```python
from build123d import *

# Parameters (mm, degrees)
SKETCH009_W                   = 120
SKETCH009_H                   = 82
PAD002_DEPTH                  = 3
SKETCH010_W                   = 16.5
SKETCH010_H                   = 3
SKETCH010_W_2                 = 11
SKETCH010_W_3                 = 3
SKETCH010_H_2                 = 18
POCKET006_DEPTH               = 293.744874
SKETCH010_MIRRORED010_2_W     = 16.5
SKETCH010_MIRRORED010_2_H     = 3
SKETCH010_MIRRORED010_2_W_2   = 11
SKETCH010_MIRRORED010_2_W_3   = 3
SKETCH010_MIRRORED010_2_H_2   = 18
POCKET006_MIRRORED010_2_DEPTH = 293.744874
SKETCH011_W                   = 15
SKETCH011_H                   = 3
POCKET007_DEPTH               = 3.001
POCKET008_DEPTH               = 3.001
SKETCH013_W                   = 2.5
SKETCH013_H                   = 4
POCKET009_DEPTH               = 3.001


with BuildPart() as part:
    # Sketch009 → Pad002 (new body)
    with BuildSketch(Plane.XZ):
        Rectangle(SKETCH009_W, SKETCH009_H)
    extrude(amount=PAD002_DEPTH)

    # Sketch010 → Pocket006 (cut, through all)
    with BuildSketch(Plane.XZ):
        with Locations((-51.75, 39.5)):
            Rectangle(SKETCH010_W, SKETCH010_H)
        with Locations((-22, 39.5)):
            Rectangle(SKETCH010_W_2, SKETCH010_H)
        with Locations((0, 39.5)):
            Rectangle(SKETCH010_W_2, SKETCH010_H)
        with Locations((-58.5, 14.5)):
            Rectangle(SKETCH010_W_3, SKETCH010_H_2)
    pocket006 = extrude(amount=POCKET006_DEPTH, mode=Mode.SUBTRACT)

    # Sketch010 Mirrored010 2 → Pocket006 Mirrored010 2 (cut, through all)
    with BuildSketch(Plane(origin=(0, 0, 0), x_dir=(-1, 0, 0), z_dir=(0, 1, 0))):
        with Locations((-51.75, 39.5)):
            Rectangle(SKETCH010_MIRRORED010_2_W, SKETCH010_MIRRORED010_2_H)
        with Locations((-22, 39.5)):
            Rectangle(SKETCH010_MIRRORED010_2_W_2, SKETCH010_MIRRORED010_2_H)
        with Locations((0, 39.5)):
            Rectangle(SKETCH010_MIRRORED010_2_W_2, SKETCH010_MIRRORED010_2_H)
        with Locations((-58.5, 14.5)):
            Rectangle(SKETCH010_MIRRORED010_2_W_3, SKETCH010_MIRRORED010_2_H_2)
    pocket006_mirrored010_2 = extrude(amount=-POCKET006_MIRRORED010_2_DEPTH, mode=Mode.SUBTRACT)

    # Mirrored011: Pocket006, Pocket006 Mirrored010 2 across Sketch010 H_Axis
    add(pocket006.mirror(Plane(origin=(0, 0, 0), x_dir=(0, -1, 0), z_dir=(0, 0, 1))), mode=Mode.SUBTRACT)
    add(pocket006_mirrored010_2.mirror(Plane(origin=(0, 0, 0), x_dir=(0, -1, 0), z_dir=(0, 0, 1))), mode=Mode.SUBTRACT)

    # Sketch011 → Pocket007 (cut, through all)
    with BuildSketch(Plane.XZ):
        with Locations((35, 3.5)):
            Rectangle(SKETCH011_W, SKETCH011_H)
        with Locations((0, 3.5)):
            Rectangle(SKETCH011_W, SKETCH011_H)
        with Locations((-35, 3.5)):
            Rectangle(SKETCH011_W, SKETCH011_H)
    extrude(amount=POCKET007_DEPTH, mode=Mode.SUBTRACT)

    # Sketch012 → Pocket008 (cut, through all)
    with BuildSketch(Plane.XZ):
        with BuildLine():
            Line((-48, 27), (8.5, 27))
            ThreePointArc((11.5, 24), (10.62132, 26.12132), (8.5, 27))
            Line((11.5, 24), (11.5, 15))
            ThreePointArc((8.5, 12), (10.62132, 12.87868), (11.5, 15))
            Line((8.5, 12), (-48, 12))
            ThreePointArc((-51, 15), (-50.12132, 12.87868), (-48, 12))
            Line((-51, 15), (-51, 24))
            ThreePointArc((-48, 27), (-50.12132, 26.12132), (-51, 24))
        make_face()
    extrude(amount=POCKET008_DEPTH, mode=Mode.SUBTRACT)

    # Sketch013 → Pocket009 (cut, through all)
    with BuildSketch(Plane.XZ):
        Polygon((60, 15.75), (53, 15.75), (53, 17), (51, 17), (51, 15.75), (47.9, 15.75), (47.9, 13.25), (51, 13.25), (51, 12), (53, 12), (53, 13.25), (60, 13.25), align=None)
        with Locations((35.5, 39)):
            Rectangle(SKETCH013_W, SKETCH013_H)
        with Locations((-35.5, 39)):
            Rectangle(SKETCH013_W, SKETCH013_H)
        with Locations((35.5, -39)):
            Rectangle(SKETCH013_W, SKETCH013_H)
        with Locations((-35.5, -39)):
            Rectangle(SKETCH013_W, SKETCH013_H)
        Polygon((60, -15.75), (53, -15.75), (53, -17), (51, -17), (51, -15.75), (47.9, -15.75), (47.9, -13.25), (51, -13.25), (51, -12), (53, -12), (53, -13.25), (60, -13.25), align=None)
        Polygon((-60, -15.75), (-53, -15.75), (-53, -17), (-51, -17), (-51, -15.75), (-47.9, -15.75), (-47.9, -13.25), (-51, -13.25), (-51, -12), (-53, -12), (-53, -13.25), (-60, -13.25), align=None)
    extrude(amount=POCKET009_DEPTH, mode=Mode.SUBTRACT)


with BuildPart() as part_1:
    # Body003 placement: moved
    add(part.part.moved(Location((0, -44.5, 0))))


solid = part_1.part
```
Design review of the part built by this model. Coordinates are the model's own, in mm. A direction names the side the tool comes from. Give positions to 0.01 mm unless a question says otherwise; leave off trailing zeros. Order: outer loops, then holes, each group sorted by start corner. A loop starts at its lowest first (then second) coordinate and runs counter-clockwise, first axis right, second up. Notation, with made-up numbers: M 43,-4.75 L 54,-4.75 A12 cw 54,8.25 Z; hole C 57.5,10 d6. An arc over 180 degrees is marked long. One line per question, with ' | ' between items. Start each with the question number.
Q1. We need section A-A (x = -22). Write out the cut boundary in (y, z).
Q2. The part is to be moulded in two halves that separate along X. For faces 4 (the face through (35, -46, 5)), 5 (the face through (-5.5, -46, -39)), 6 (the face through (-57, -46, -20)), 7 (the face through (49, -46, -15.75)), say which applies: +X half, -X half, draft (parallel to the pull), parting line (faces both ways), or undercut.
Q3. Machinability: for faces 1 (the face through (34.25, -46, 39)), 2 (the face through (-47.9, -46, -15)), 3 (the face through (47.9, -46, 15)), which of the approach directions +Z, -Z, +X, -X, +Y, -Y give a long, thin tool a straight path to every point of the face, cutting with its end or side? Answer none if there is none.
Q4. For L1, parallel to Z at x = -31.5, y = -45.5; L2, parallel to Z at x = -3, y = -47.35; L3, parallel to Z at x = 40.5, y = -46.3, list the stretches that pass through material, from the lowest coordinate up. Write a range as [from, to].
Q5. We need section B-B (y = -45). State how many separate pieces and enclosed holes the cut face has, plus the area to 3 significant figures.
Q6. For pin 1 Ø1.5 at (y, z) = (-46, 39) entering from -X; pin 2 Ø1 at (y, z) = (-46, -16.5) entering from +X; pin 3 Ø0.6 at (y, z) = (-46.5, 12.5) entering from -X, all flat-tipped, find the tip position at first contact; note any pin that passes through.
Returned:
1) outline: M -47.5,-38 L -44.5,-38 L -44.5,12 L -47.5,12 Z; M -47.5,27 L -44.5,27 L -44.5,38 L -47.5,38 Z
2) face 4: undercut | face 5: undercut | face 6: -X half | face 7: draft
3) face 1: +Z, +Y, -Y | face 2: -X, +Y, -Y | face 3: +X, +Y, -Y
4) L1: [-41, 2], [5, 12], [27, 41] | L2: [-38, 2], [5, 12], [27, 38] | L3: [-41, 2], [5, 41]
5) separate pieces: 1 | enclosed holes: 4 | area: 8,040 mm2
6) pin 1: x = -43.5 | pin 2: x = 57 | pin 3: x = -57
